Can you work these out from the model? Positions are in its coordinate system, mm. Round coordinates to 2 decimals unless told otherwise and drop trailing zeros. Loops run counter-clockwise (first coordinate to the right, second up) from the corner with the lowest first, then second, coordinate; pieces in that order, holes last. Notation, with made-up numbers: (-37.75, -21) -> (11.25, -21) arc R23 cw to (11.25, 9) -> close; hole circle Ø3 at (-37.5, 19). An arc over 180 degrees is marked (long way). Use a Markdown table: item, result.
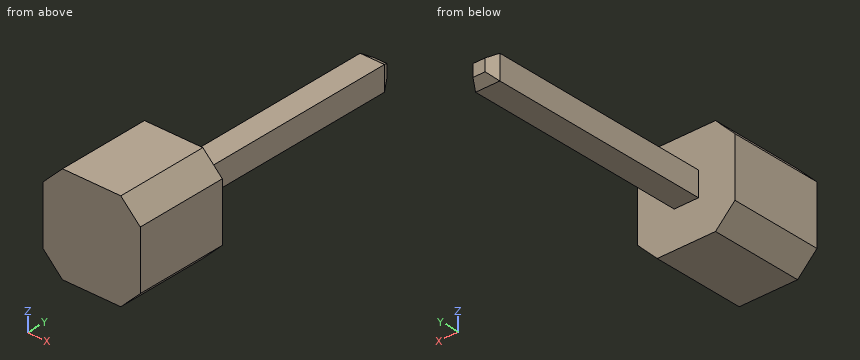
from build123d import *
from OCP.BRepFilletAPI import BRepFilletAPI_MakeChamfer

# Parameters (mm, degrees)
SKETCH1_W           = 2.54
SKETCH1_H           = 2.54
BOSS_EXTRUDE1_DEPTH = 2.413
CHAMFER1_SIZE       = 0.508
SKETCH2_W           = 0.635
SKETCH2_H           = 0.635
BOSS_EXTRUDE2_DEPTH = 6.096
CHAMFER2_SIZE       = 0.254
CHAMFER2_SIZE2      = 0.158716815


with BuildPart() as part:
    # Sketch1 → Boss-Extrude1 (new body)
    with BuildSketch(Plane(origin=(0, 0, 0), x_dir=(1, 0, 0), z_dir=(0, 1, 0))):
        Rectangle(SKETCH1_W, SKETCH1_H)
    extrude(amount=BOSS_EXTRUDE1_DEPTH)

    # Chamfer1
    chamfer1_edges = [part.edges().sort_by_distance(p)[0] for p in [
        (1.27, 1.2065, 1.27),
        (-1.27, 1.2065, 1.27),
        (-1.27, 1.2065, -1.27),
        (1.27, 1.2065, -1.27),
    ]]
    chamfer(chamfer1_edges, length=CHAMFER1_SIZE)

    # Sketch2 → Boss-Extrude2 (add)
    with BuildSketch(Plane(origin=(0, 2.413, 0), x_dir=(1, 0, 0), z_dir=(0, 1, 0))):
        Rectangle(SKETCH2_W, SKETCH2_H)
    extrude(amount=BOSS_EXTRUDE2_DEPTH)

    # Chamfer2: one chamfer whose edges measure the first distance from different faces: ONE call of the kernel's chamfer builder (chamfer() names one face for all edges)
    chamfer2_edges_1 = [part.edges().sort_by_distance(p)[0] for p in [
        (0.3175, 8.509, 0),
    ]]
    chamfer2_side_1 = [part.faces().sort_by_distance(p)[0] for p in [
        (0.3175, 5.461, 0),
    ]]
    chamfer2_edges_2 = [part.edges().sort_by_distance(p)[0] for p in [
        (0, 8.509, -0.3175),
    ]]
    chamfer2_side_2 = [part.faces().sort_by_distance(p)[0] for p in [
        (0, 5.461, -0.3175),
    ]]
    chamfer2_edges_3 = [part.edges().sort_by_distance(p)[0] for p in [
        (-0.3175, 8.509, 0),
    ]]
    chamfer2_side_3 = [part.faces().sort_by_distance(p)[0] for p in [
        (-0.3175, 5.461, 0),
    ]]
    chamfer2_edges_4 = [part.edges().sort_by_distance(p)[0] for p in [
        (0, 8.509, 0.3175),
    ]]
    chamfer2_side_4 = [part.faces().sort_by_distance(p)[0] for p in [
        (0, 5.461, 0.3175),
    ]]
    chamfer2 = BRepFilletAPI_MakeChamfer(part.part.solid().wrapped)
    for e in chamfer2_edges_1:
        chamfer2.Add(CHAMFER2_SIZE, CHAMFER2_SIZE2, e.wrapped, chamfer2_side_1[0].wrapped)  # the first distance lies on this face
    for e in chamfer2_edges_2:
        chamfer2.Add(CHAMFER2_SIZE, CHAMFER2_SIZE2, e.wrapped, chamfer2_side_2[0].wrapped)  # the first distance lies on this face
    for e in chamfer2_edges_3:
        chamfer2.Add(CHAMFER2_SIZE, CHAMFER2_SIZE2, e.wrapped, chamfer2_side_3[0].wrapped)  # the first distance lies on this face
    for e in chamfer2_edges_4:
        chamfer2.Add(CHAMFER2_SIZE, CHAMFER2_SIZE2, e.wrapped, chamfer2_side_4[0].wrapped)  # the first distance lies on this face
    add(Compound.cast(chamfer2.Shape()), mode=Mode.REPLACE)


solid = part.part
1. I want a section at B-B (y = 1.25). Please give me the cut outline in (x, z), plus the area to 3 significant figures.
Answer sheet:
| item | result |
|---|---|
| outline | (-1.27, -0.76) -> (-0.76, -1.27) -> (0.76, -1.27) -> (1.27, -0.76) -> (1.27, 0.76) -> (0.76, 1.27) -> (-0.76, 1.27) -> (-1.27, 0.76) -> close |
| area | 5.94 mm² |
2. I want a section at C-C (x = 0.45). Please give me the cut outline in (y, z), plus the area to 3 significant figures.
Answer sheet:
| item | result |
|---|---|
| outline | (0, -1.27) -> (2.41, -1.27) -> (2.41, 1.27) -> (0, 1.27) -> close |
| area | 6.13 mm² |
3. I need wall thicknesses on line 1 (Y direction, x = 0.85, z = -0.1); line 2 (X direction, y = 7, z = 0.15). Which ranges of each line are inside material? Lowest first, please.
Answer sheet:
| item | result |
|---|---|
| line 1 | y = 0 to 2.41 |
| line 2 | x = -0.32 to 0.32 |
4. I want a section at D-D (z = 0.5). Please give me the cut outline in (x, y).
Answer sheet:
| item | result |
|---|---|
| outline | (-1.27, 0) -> (1.27, 0) -> (1.27, 2.41) -> (-1.27, 2.41) -> close |
5. Will these pins go through, and if not, where does the flat tip stop? pin 1 Ø0.5 at (x, y) = (0, 7) entering from -Z; pin 2 Ø1 at (x, z) = (0, -1) entering from +Y; pin 3 Ø1 at (y, z) = (3, 0) entering from -X.
Answer sheet:
| item | result |
|---|---|
| pin 1 | stops at z = -0.32 |
| pin 2 | stops at y = 2.41 |
| pin 3 | stops at x = -0.32 |
